Source: CAD feature listing. Evaluate the final solid. Frame: model axes, mm. A direction names the side the tool comes from. Round coordinates to 2 decimals unless told otherwise and drop trailing zeros. Order: outer loops, then holes, each group sorted by start corner. A loop starts at its lowest first (then second) coordinate and runs counter-clockwise, first axis right, second up. Notation, with made-up numbers: (44.5, 25.5) -> (70.5, 25.5) arc R25 cw to (70.5, 44.5) -> close; hole circle Ø10 at (46, -14.5). An arc over 180 degrees is marked (long way). Answer as CSV lines item,"result".
from build123d import *

# Parameters (mm, degrees)
SKETCH1_W           = 18
SKETCH1_H           = 18
BOSS_EXTRUDE2_DEPTH = 3
SKETCH2_W           = 3
SKETCH2_H           = 18
BOSS_EXTRUDE3_DEPTH = 15
SKETCH3_W           = 3
SKETCH3_H           = 18
BOSS_EXTRUDE4_DEPTH = 15
SKETCH5_W           = 11.999914095
SKETCH5_H           = 2.5
BOSS_EXTRUDE5_DEPTH = 15
FILLET1_R           = 2
FILLET2_R           = 2
SKETCH6_R           = 3
CUT_EXTRUDE1_DEPTH  = 19


with BuildPart() as part:
    # Sketch1 → Boss-Extrude2 (new body)
    with BuildSketch(Plane.XY):
        with Locations((9, 9)):
            Rectangle(SKETCH1_W, SKETCH1_H)
    extrude(amount=BOSS_EXTRUDE2_DEPTH)

    # Sketch2 → Boss-Extrude3 (add)
    with BuildSketch(Plane.XY.offset(3)):
        with Locations((16.499914095, 9)):
            Rectangle(SKETCH2_W, SKETCH2_H)
    extrude(amount=BOSS_EXTRUDE3_DEPTH)

    # Sketch3 → Boss-Extrude4 (add)
    with BuildSketch(Plane.XY.offset(3)):
        with Locations((1.5, 9)):
            Rectangle(SKETCH3_W, SKETCH3_H)
    extrude(amount=BOSS_EXTRUDE4_DEPTH)

    # Sketch5 → Boss-Extrude5 (add)
    with BuildSketch(Plane.XY.offset(3)):
        with Locations((8.999957048, 1.25)):
            Rectangle(SKETCH5_W, SKETCH5_H)
    extrude(amount=BOSS_EXTRUDE5_DEPTH)

    # Fillet1
    fillet1_edges = [part.edges().sort_by_distance(p)[0] for p in [
        (0, 9, 0),
    ]]
    fillet(fillet1_edges, radius=FILLET1_R)

    # Fillet2
    fillet2_edges = [part.edges().sort_by_distance(p)[0] for p in [
        (18, 9, 0),
    ]]
    fillet(fillet2_edges, radius=FILLET2_R)

    # Sketch6 → Cut-Extrude1 (cut, through all)
    with BuildSketch(Plane.XZ):
        with Locations((8.999957047, 12)):
            Circle(SKETCH6_R)
    extrude(amount=-CUT_EXTRUDE1_DEPTH, mode=Mode.SUBTRACT)


solid = part.part
1. Mould query, pull axis X, two halves, no side actions, for faces 1 (the flat face through (3, 10, 10)), 2 (the cylindrical face through (0.57, 9.13, 0.6)), 3 (the cylindrical face through (17.4, 9.13, 0.57)), 4 (the flat face through (9, 9, 0)). Classes: released by +X, released by -X, zero draft, split by the parting line, or undercut.
Results below:
face 1,"undercut"
face 2,"released by -X"
face 3,"released by +X"
face 4,"zero draft"
2. Section query B-B on z = 12. Return loops of the section in (x, y).
Results below:
outline,"(0, 0) -> (6, 0) -> (6, 2.5) -> (3, 2.5) -> (3, 18) -> (0, 18) -> close; (12, 0) -> (18, 0) -> (18, 18) -> (15, 18) -> (15, 2.5) -> (12, 2.5) -> close"
3. Line query: L1, parallel to X at y = 12.75, z = 10; L2, parallel to Z at x = 8, y = 12; L3, parallel to Z at x = 11.5, y = 2. Output: solid intervals per line, ascending. Write a range as [from, to].
Results below:
L1,"[0, 3], [15, 18]"
L2,"[0, 3]"
L3,"[0, 10.34], [13.66, 18]"
4. Section query C-C on x = 7.25. Return loops of the section in (y, z), and give its area (3 significant figures).
Results below:
outline,"(0, 0) -> (18, 0) -> (18, 3) -> (2.5, 3) -> (2.5, 9.56) -> (0, 9.56) -> close; (0, 14.44) -> (2.5, 14.44) -> (2.5, 18) -> (0, 18) -> close"
area,"79.3 mm2"
5. Pin query (flat end, axial travel): pin 1 (9.5 mm diameter, centred on x = 10, z = 7.5, fed in from +Y); pin 2 (2 mm diameter, centred on x = 13.5, y = 14.5, fed in from +Z); pin 3 (5.5 mm diameter, centred on x = 9, z = 12, fed in from -Y); pin 4 (1 mm diameter, centred on x = 12.5, z = 6.5, fed in from +Y). Return the tip coordinate at first contact, or that it passes through.
Results below:
pin 1,"y = 18"
pin 2,"z = 3"
pin 3,"through"
pin 4,"y = 2.5"
6. Reachability of faces 5 (the flat face through (9, 0, 7)), 6 (the flat face through (8.9, 2.5, 8.7)) from +Z, -Z, +X, -X, +Y, -Y: full face, straight path, thin tool, end or side. Return the list, or none.
Results below:
face 5,"+Z, -Z, +X, -X, -Y"
face 6,"+Z, +Y"
7. Section query D-D on x = 4. Return loops of the section in (y, z).
Results below:
outline,"(0, 0) -> (18, 0) -> (18, 3) -> (2.5, 3) -> (2.5, 18) -> (0, 18) -> close"
